from build123d import *

# Parameters (mm, degrees)
BOSS_EXTRUDE1_DEPTH = 6
BOSS_EXTRUDE2_DEPTH = 3.8
SKETCH3_R           = 1.4
CUT_EXTRUDE1_DEPTH  = 13.009524001


with BuildPart() as part:
    # Sketch1 → Boss-Extrude1 (new body)
    with BuildSketch(Plane(origin=(0, 0, 0), x_dir=(0, 1, 0), z_dir=(0, 0, 1))):
        with BuildLine():
            Line((-4.4, -3.077119877), (-4.4, 3.077119877))
            ThreePointArc((-4.4, 3.077119877), (0, 5.369233347), (4.4, 3.077119877))
            Line((4.4, 3.077119877), (4.4, -3.077119877))
            ThreePointArc((4.4, -3.077119877), (0, -5.369233347), (-4.4, -3.077119877))
        make_face()
        with BuildLine():
            ThreePointArc((-1.9, -2.15), (0, -2.869233347), (1.9, -2.15))
            Line((1.9, -2.15), (1.9, 2.15))
            ThreePointArc((1.9, 2.15), (0, 2.869233347), (-1.9, 2.15))
            Line((-1.9, 2.15), (-1.9, -2.15))
        make_face(mode=Mode.SUBTRACT)
    extrude(amount=BOSS_EXTRUDE1_DEPTH)

    # Sketch2 → Boss-Extrude2 (add)
    with BuildSketch(Plane.XY.offset(6)):
        with BuildLine():
            Line((-3.728872107, -0.818543418), (-3.728872107, 0.981456582))
            Line((-3.728872107, 0.981456582), (-2.728872107, 0.981456582))
            ThreePointArc((-2.728872107, 0.981456582), (2.898733684, -0.085691473), (-2.782083153, -0.818543418))
            Line((-2.782083153, -0.818543418), (-3.728872107, -0.818543418))
        make_face()
    extrude(amount=BOSS_EXTRUDE2_DEPTH)

    # Sketch3 → Cut-Extrude1 (cut, through all)
    with BuildSketch(Plane.XY.offset(9.8)):
        Circle(SKETCH3_R)
    extrude(amount=-CUT_EXTRUDE1_DEPTH, mode=Mode.SUBTRACT)


solid = part.part
Design review of the part built by this model. Coordinates are the model's own, in mm. A direction names the side the tool comes from. Round coordinates to 2 decimals unless told otherwise and drop trailing zeros. Write each loop counter-clockwise with the first axis right and the second up, starting at its lowest first coordinate (ties: lowest second). Pieces come first, ordered by that corner, then holes. Notation, with made-up numbers: (48, 79) -> (71, 79) arc R26 cw to (71, 117) -> close; hole circle Ø7 at (-7.75, -33). An arc over 180 degrees is marked (long way). One line per item, written item: value. Start each with the question number.
Q1. Add section D-D (x = -3.5). Give the boundary of the cut face in (y, z), then the cut area to 3 significant figures.
Q2. To check wall thickness, follow probe 1 along Y at (x, z) = (0, 8.8); probe 2 along Y at (x, z) = (0, 3); probe 3 along X at (y, z) = (0, 3). State the ranges of each line that lie inside material, in increasing order.
Q3. Add section B-B (y = 0). Give the boundary of the cut face in (x, z), then the cut area to 3 significant figures.
Q4. Insertion check: P1, Ø4, axis at y = 3, z = 5, coming from the -X side; P2, Ø2.5, axis at x = 0, y = 0, coming from the +Z side. Each pin has a flat end and moves straight along its axis. Give the tip position at first contact, or say it passes through.
Q5. Add section C-C (z = 2). Give the boundary of the cut face in (x, y), then the cut area to 3 significant figures.
Q6. Add section A-A (x = 0). Give the boundary of the cut face in (y, z), then the cut area to 3 significant figures.
Q7. Tool access review of faces 4 (the face through (-3, -0.819, 8)), 5 (the face through (-3, 0.981, 8)), 6 (the face through (2.9, 0, 7.9)), 7 (the face through (0, -1.9, 3)): name each direction out of +Z, -Z, +X, -X, +Y, -Y from which nothing blocks a thin tool from reaching the whole face with its end or side.
Q8. The part is to be moulded in two halves that separate along X. For faces 1 (the face through (-3.729, 0, 8)), 2 (the face through (1.3, 0.9, 6)), 3 (the face through (0, 3, 0)), say which applies: pulls with the +X half, pulls with the -X half, needs draft (parallel to the pull), parting line crosses it, or undercut.
Response:
1. outline: (-4.07, 0) -> (4.07, 0) -> (4.07, 6) -> (0.98, 6) -> (0.98, 9.8) -> (-0.82, 9.8) -> (-0.82, 6) -> (-4.07, 6) -> close
1. area: 55.7 mm^2
2. probe 1: y = -2.9 to -1.4, 1.4 to 2.9
2. probe 2: y = -4.4 to -1.9, 1.9 to 4.4
2. probe 3: x = -5.37 to -2.87, 2.87 to 5.37
3. outline: (-5.37, 0) -> (-2.87, 0) -> (-2.87, 6) -> (-1.4, 6) -> (-1.4, 9.8) -> (-3.73, 9.8) -> (-3.73, 6) -> (-5.37, 6) -> close; (1.4, 6) -> (2.87, 6) -> (2.87, 0) -> (5.37, 0) -> (5.37, 6) -> (2.9, 6) -> (2.9, 9.8) -> (1.4, 9.8) -> close
3. area: 44.5 mm^2
4. P1: stops at x = -5.28
4. P2: passes through
5. outline: (-3.08, -4.4) -> (3.08, -4.4) arc R5.37 ccw to (3.08, 4.4) -> (-3.08, 4.4) arc R5.37 ccw to start; hole (-2.15, -1.9) -> (2.15, -1.9) arc R2.87 ccw to (2.15, 1.9) -> (-2.15, 1.9) arc R2.87 ccw to start
5. area: 62.4 mm^2
6. outline: (-4.4, 0) -> (-1.9, 0) -> (-1.9, 6) -> (-1.4, 6) -> (-1.4, 9.8) -> (-2.9, 9.8) -> (-2.9, 6) -> (-4.4, 6) -> close; (1.4, 6) -> (1.9, 6) -> (1.9, 0) -> (4.4, 0) -> (4.4, 6) -> (2.9, 6) -> (2.9, 9.8) -> (1.4, 9.8) -> close
6. area: 41.4 mm^2
7. face 4: +Z, -X, -Y
7. face 5: +Z, -X, +Y
7. face 6: +Z
7. face 7: -Z
8. face 1: pulls with the -X half
8. face 2: undercut
8. face 3: needs draft
